Check sheet for the modelled part. Datum: model origin and axes. Units: mm. A direction names the side the tool comes from. Round coordinates to 2 decimals unless told otherwise and drop trailing zeros. Loops run counter-clockwise (first coordinate to the right, second up) from the corner with the lowest first, then second, coordinate; pieces in that order, holes last. Notation, with made-up numbers: M 49,46 L 100,46 A11 ccw 100,50 Z; hole C 58.25,76 d3. An arc over 180 degrees is marked long. Write item = value, one per line. Start each with the question number.
(1) Set-up check for faces 5 (the face through (-1, -3, 2)), 6 (the face through (8.953, -0.057, 1.014)), 7 (the face through (12, 0, 10.096)): record each of +Z, -Z, +X, -X, +Y, -Y from which the full face is reachable in a straight line by a thin tool's end or side.
(2) Scan lines: L1, parallel to Z at x = 4, y = -6.25; L2, parallel to Y at x = 9, z = 18.5. Record each from-to range of solid material in increasing order. Write a range as from..to.
(3) Mould release check, pull along X, two halves, no side actions. Record for faces 1 (the face through (0, -2.604, 1)), 2 (the face through (12.1, -0.59, 0.57)), 3 (the face through (12, 0, 15.304)), 4 (the face through (2.604, 12, 13)): pulls with the +X half, pulls with the -X half, needs draft (parallel to the pull), parting line crosses it, or undercut.
(4) Cross-section at B-B on x = -5.5. Record the boundary of the cut face in (y, z).
(5) Cross-section at A-A on y = 0. Record the boundary of the cut face in (x, z).
(6) Cross-section at C-C on x = 0. Record the boundary of the cut face in (y, z), plus the area to 3 significant figures.
(7) Go/stop test with flat-tipped pins: P1, Ø6, axis at x = 3, z = 16.5, coming from the -Y side; P2, Ø12, axis at y = 2.5, z = 22.5, coming from the -X side; P3, Ø0.6, axis at x = 0, z = 0.5, coming from the +Y side. Record where each tip stops, or that it passes through.
(8) Cross-section at D-D on z = 23.25. Record the boundary of the cut face in (x, y).
from build123d import *

# Parameters (mm, degrees)
SKETCH014_W     = 25.4
SKETCH014_H     = 25.4
PAD007_DEPTH    = 25.4
SKETCH015_W     = 23.4
SKETCH015_H     = 23.4
POCKET005_DEPTH = 23.4
POCKET006_DEPTH = 2.001
POCKET007_DEPTH = 2.001
POCKET008_DEPTH = 2.001
FILLET005_R     = 2
FILLET006_R     = 0.5


with BuildPart() as part:
    # Sketch014 → Pad007 (new body)
    with BuildSketch(Plane.XY):
        Rectangle(SKETCH014_W, SKETCH014_H)
    extrude(amount=PAD007_DEPTH)

    # Sketch015 (on Face6 of Pad007) → Pocket005 (cut)
    with BuildSketch(Plane.XY.offset(25.4)):
        with Locations((-1, -1)):
            Rectangle(SKETCH015_W, SKETCH015_H)
    extrude(amount=-POCKET005_DEPTH, mode=Mode.SUBTRACT)

    # Sketch016 (on Face7 of Pocket005) → Pocket006 (cut, through all)
    with BuildSketch(Plane.XY.offset(2)):
        with BuildLine():
            ThreePointArc((-6.35, 2.6035), (-8.9535, 0), (-6.35, -2.6035))
            Line((-6.35, -2.6035), (6.35, -2.6035))
            ThreePointArc((6.35, -2.6035), (8.9535, 0), (6.35, 2.6035))
            Line((6.35, 2.6035), (-6.35, 2.6035))
        make_face()
    extrude(amount=-POCKET006_DEPTH, mode=Mode.SUBTRACT)

    # Sketch017 (on Face6 of Pocket006) → Pocket007 (cut, through all)
    with BuildSketch(Plane(origin=(10.7, 0, 0), x_dir=(0, -1, 0), z_dir=(-1, 0, 0))):
        with BuildLine():
            ThreePointArc((-6.35, 15.3035), (-8.9535, 12.7), (-6.35, 10.0965))
            Line((-6.35, 10.0965), (6.35, 10.0965))
            ThreePointArc((6.35, 10.0965), (8.9535, 12.7), (6.35, 15.3035))
            Line((6.35, 15.3035), (-6.35, 15.3035))
        make_face()
    extrude(amount=-POCKET007_DEPTH, mode=Mode.SUBTRACT)

    # Sketch018 (on Face17 of Pocket007) → Pocket008 (cut, through all)
    with BuildSketch(Plane.XZ.offset(-10.7)):
        with BuildLine():
            ThreePointArc((2.6035, 19.05), (0, 21.6535), (-2.6035, 19.05))
            Line((-2.6035, 19.05), (-2.6035, 6.35))
            ThreePointArc((-2.6035, 6.35), (0, 3.7465), (2.6035, 6.35))
            Line((2.6035, 6.35), (2.6035, 19.05))
        make_face()
    extrude(amount=-POCKET008_DEPTH, mode=Mode.SUBTRACT)

    # Fillet005
    fillet005_edges = [part.edges().sort_by_distance(p)[0] for p in [
        (12.7, 12.7, 12.7),
        (0, 12.7, 0),
        (12.7, 0, 0),
    ]]
    fillet(fillet005_edges, radius=FILLET005_R)

    # Fillet006
    fillet006_edges = [part.edges().sort_by_distance(p)[0] for p in [
        (-1, -12.7, 0),
        (12.114214, -12.7, 0.585786),
        (-12.7, -12.7, 1),
        (12.7, -12.7, 13.7),
        (-1, -12.7, 2),
        (11.7, -12.7, 25.4),
        (10.7, -12.7, 13.7),
        (-1, 12.7, 25.4),
        (12.114214, 12.114214, 25.4),
        (-12.7, 11.7, 25.4),
        (12.7, -1, 25.4),
        (-1, 10.7, 25.4),
        (10.7, -1, 25.4),
        (-12.7, -1, 0),
        (-12.7, 12.114214, 0.585786),
        (-12.7, 12.7, 13.7),
        (-12.7, -1, 2),
        (-12.7, 10.7, 13.7),
    ]]
    fillet(fillet006_edges, radius=FILLET006_R)


solid = part.part
Result:
q1.face_5 = +Z, -X, -Y
q1.face_6 = +Z, -Z
q1.face_7 = +X, -X
q2.L1 = 0..2
q2.L2 = 10.7..12.7
q3.face_1 = undercut
q3.face_2 = pulls with the +X half
q3.face_3 = needs draft
q3.face_4 = undercut
q4.outline = M -12.7,0.5 A0.5 ccw -12.2,0 L -2.6,0 L -2.6,2 L -12.2,2 A0.5 ccw -12.7,1.5 Z; M 2.6,0 L 10.7,0 A2 ccw 12.7,2 L 12.7,24.9 A0.5 ccw 12.2,25.4 L 11.2,25.4 A0.5 ccw 10.7,24.9 L 10.7,2 L 2.6,2 Z
q5.outline = M -12.7,0.5 A0.5 ccw -12.2,0 L -8.95,0 L -8.95,2 L -12.2,2 A0.5 ccw -12.7,1.5 Z; M 8.95,0 L 10.7,0 A2 ccw 12.7,2 L 12.7,10.1 L 10.7,10.1 L 10.7,2 L 8.95,2 Z; M 10.7,15.3 L 12.7,15.3 L 12.7,24.9 A0.5 ccw 12.2,25.4 L 11.2,25.4 A0.5 ccw 10.7,24.9 Z
q6.outline = M -12.7,0.5 A0.5 ccw -12.2,0 L -2.6,0 L -2.6,2 L -12.2,2 A0.5 ccw -12.7,1.5 Z; M 2.6,0 L 10.7,0 A2 ccw 12.7,2 L 12.7,3.75 L 10.7,3.75 L 10.7,2 L 2.6,2 Z; M 10.7,21.65 L 12.7,21.65 L 12.7,24.9 A0.5 ccw 12.2,25.4 L 11.2,25.4 A0.5 ccw 10.7,24.9 Z
q6.area = 50.3 mm^2
q7.P1 = 10.7
q7.P2 = 10.7
q7.P3 = 12.3
q8.outline = M -12.7,11.2 A0.5 ccw -12.2,10.7 L 10.7,10.7 L 10.7,-12.2 A0.5 ccw 11.2,-12.7 L 12.2,-12.7 A0.5 ccw 12.7,-12.2 L 12.7,10.7 A2 ccw 10.7,12.7 L -12.2,12.7 A0.5 ccw -12.7,12.2 Z
